Read the model definition and answer for the solid it produces. Units are mm, in the model's axes. Face numbers are marked on the shaded views. A direction names the side the tool comes from. Coordinates: 2 decimals unless noted, no trailing zeros. Write each loop counter-clockwise with the first axis right and the second up, starting at its lowest first coordinate (ties: lowest second). Pieces come first, ordered by that corner, then holes. Notation, with made-up numbers: (-2.75, -26) - (49.25, -26) arc R20 ccw to (49.25, 4) - close; hole circle Ø2 at (-18, 30.5). An arc over 180 degrees is marked (long way). Use a Markdown table: item, result.
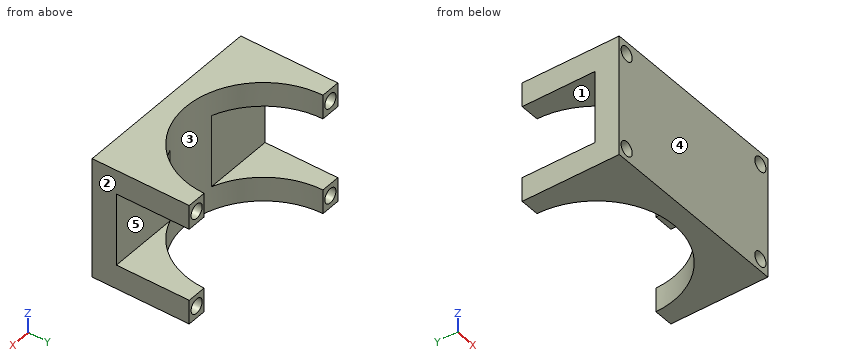
from build123d import *

# Parameters (mm, degrees)
CROQUIS1_W              = 40
CROQUIS1_H              = 25
SALIENTE_EXTRUIR1_DEPTH = 20
CROQUIS2_R              = 16
CORTAR_EXTRUIR1_DEPTH   = 26
CROQUIS3_R              = 1.5
CORTAR_EXTRUIR2_DEPTH   = 21
CROQUIS4_W              = 15
CROQUIS4_H              = 15
CORTAR_EXTRUIR3_DEPTH   = 41


with BuildPart() as part:
    # Croquis1 → Saliente-Extruir1 (new body)
    with BuildSketch(Plane(origin=(0, 0, 0), x_dir=(1, 0, 0), z_dir=(0, 1, 0))):
        with Locations((20, 12.5)):
            Rectangle(CROQUIS1_W, CROQUIS1_H)
    extrude(amount=SALIENTE_EXTRUIR1_DEPTH)

    # Croquis2 → Cortar-Extruir1 (cut, through all)
    with BuildSketch(Plane.XY):
        with Locations((20, 20)):
            Circle(CROQUIS2_R)
    extrude(amount=-CORTAR_EXTRUIR1_DEPTH, mode=Mode.SUBTRACT)

    # Croquis3 → Cortar-Extruir2 (cut, through all)
    with BuildSketch(Plane(origin=(0, 20, 0), x_dir=(1, 0, 0), z_dir=(0, 1, 0))):
        with Locations((2, 2.5)):
            Circle(CROQUIS3_R)
        with Locations((2, 22.5)):
            Circle(CROQUIS3_R)
        with Locations((38, 2.5)):
            Circle(CROQUIS3_R)
        with Locations((38, 22.5)):
            Circle(CROQUIS3_R)
    extrude(amount=-CORTAR_EXTRUIR2_DEPTH, mode=Mode.SUBTRACT)

    # Croquis4 → Cortar-Extruir3 (cut, through all)
    with BuildSketch(Plane(origin=(40, 0, 0), x_dir=(0, 0, -1), z_dir=(1, 0, 0))):
        with Locations((12.5, 12.5)):
            Rectangle(CROQUIS4_W, CROQUIS4_H)
    extrude(amount=-CORTAR_EXTRUIR3_DEPTH, mode=Mode.SUBTRACT)


solid = part.part
(1) A cutting plane is placed at A-A, the plane x = 2. Write down the section's boundary in (y, z).
Report:
| item | result |
|---|---|
| outline | (0, -25) - (20, -25) - (20, -24) - (0, -24) - close; (0, -21) - (20, -21) - (20, -20) - (5, -20) - (5, -5) - (20, -5) - (20, -4) - (0, -4) - close; (0, -1) - (20, -1) - (20, 0) - (0, 0) - close |
(2) For the marked faces 4 and 5, determine the directions among +Z, -Z, +X, -X, +Y, -Y from which every point of the face is accessible in a straight line to the end or side of a thin tool.
Report:
| item | result |
|---|---|
| face 4 | +Z, -Z, +X, -X, -Y |
| face 5 | +X, -X, +Y |
(3) Each of these flat-tipped pins is pushed along its axis until it touches: P1, Ø7, axis at x = 9, z = -13.5, coming from the +Y side; P2, Ø1.8, axis at x = 38, z = -2.5, coming from the -Y side. Where does it stop, or does it pass through?
Report:
| item | result |
|---|---|
| P1 | stops at y = 5 |
| P2 | passes through |
(4) A cutting plane is placed at B-B, the plane z = -2.5. Write down the section's boundary in (x, y).
Report:
| item | result |
|---|---|
| outline | (0, 0) - (0.5, 0) - (0.5, 20) - (0, 20) - close; (3.5, 0) - (36.5, 0) - (36.5, 20) - (36, 20) arc R16 cw to (4, 20) - (3.5, 20) - close; (39.5, 0) - (40, 0) - (40, 20) - (39.5, 20) - close |
(5) A cutting plane is placed at C-C, the plane y = 8.75. Write down the section's boundary in (x, z), and give its area (3 significant figures).
Report:
| item | result |
|---|---|
| outline | (0, -25) - (8.62, -25) - (8.62, -20) - (0, -20) - close; (0, -5) - (8.62, -5) - (8.62, 0) - (0, 0) - close; (31.38, -25) - (40, -25) - (40, -20) - (31.38, -20) - close; (31.38, -5) - (40, -5) - (40, 0) - (31.38, 0) - close; hole circle Ø3 at (2, -22.5); hole circle Ø3 at (2, -2.5); hole circle Ø3 at (38, -22.5); hole circle Ø3 at (38, -2.5) |
| area | 144 mm² |
(6) The mould has two halves that part along X. Classify the marked faces 1, 2 and 3: pulls with the +X half, pulls with the -X half, needs draft (parallel to the pull), parting line crosses it, or undercut.
Report:
| item | result |
|---|---|
| face 1 | needs draft |
| face 2 | pulls with the +X half |
| face 3 | undercut |
(7) Straight lines are drawn through the part: L1, parallel to Z at x = 38, y = 13.25; L2, parallel to X at y = 3.75, z = -23.25; L3, parallel to X at y = 15.5, z = -22.5. For each, find the intervals that lie inside material, in ascending order.
Report:
| item | result |
|---|---|
| L1 | z = -25 to -24, -21 to -20, -5 to -4, -1 to 0 |
| L2 | x = 0 to 0.7, 3.3 to 36.7, 39.3 to 40 |
| L3 | x = 0 to 0.5, 3.5 to 4.65, 35.35 to 36.5, 39.5 to 40 |
(8) A cutting plane is placed at D-D, the plane y = 3.5. Write down the section's boundary in (x, z).
Report:
| item | result |
|---|---|
| outline | (0, -25) - (40, -25) - (40, 0) - (0, 0) - close; hole circle Ø3 at (2, -22.5); hole circle Ø3 at (2, -2.5); hole circle Ø3 at (38, -22.5); hole circle Ø3 at (38, -2.5) |
